Answer from the drawing. Dimensions are ordinates in mm from the lowest x, y and z of the part. Coordinates: 2 decimals unless noted, no trailing zeros.
(1) Find the intervals of material crossed by probe 1 along Y at (x, z) = (388, 19.5), in increasing order.
(2) Section B-B on y = 10.75 is taken. State how many separate pieces and enclosed holes the cut face has, then the cut area to 3 significant figures.
(3) Given pin 1 (7.5 mm diameter, centred on x = 373.5, z = 22.5, fed in from +Y); pin 2 (1.5 mm diameter, centred on x = 205, z = 100, fed in from -Y); pin 3 (7.5 mm diameter, centred on x = 30, z = 165, fed in from +Y), each flat-ended and moving along its own axis, determine where each tip first touches the part or whether it passes through.
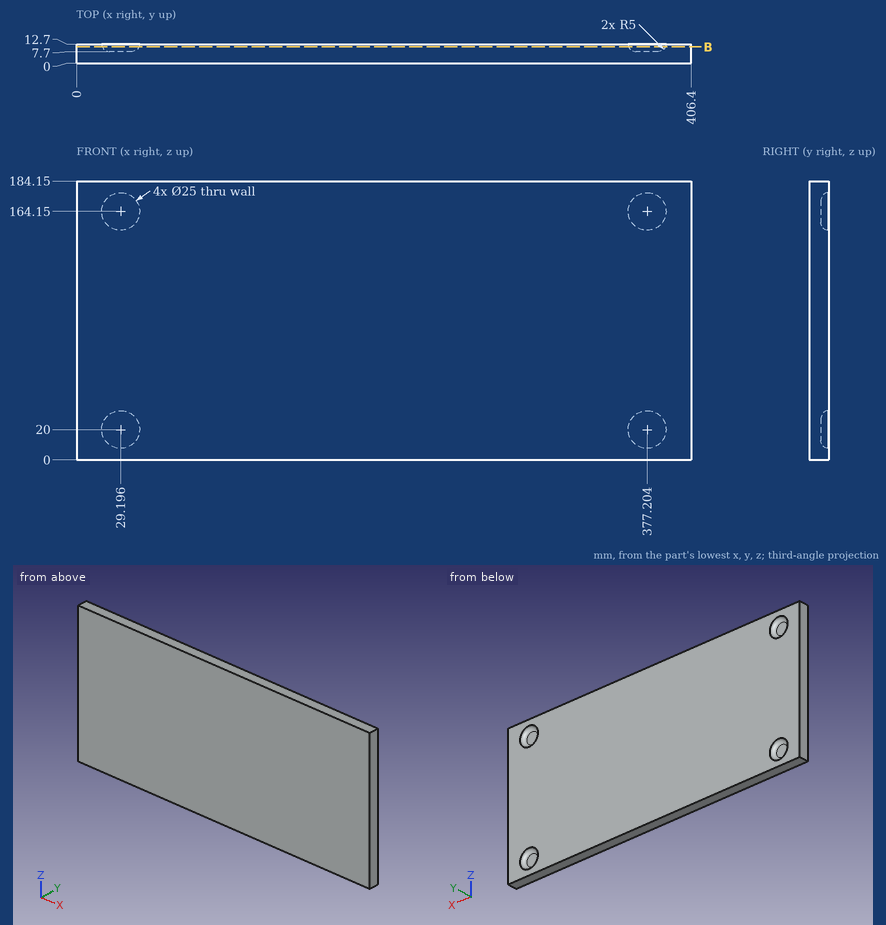
Response:
1. probe 1: y = 0 to 8.95
2. separate pieces: 1
2. enclosed holes: 4
2. area: 73,000 mm2
3. pin 1: stops at y = 7.75
3. pin 2: stops at y = 0
3. pin 3: stops at y = 7.7
